Here's how the part is built. I have some questions about the finished solid (model axes, mm). A direction names the side the tool comes from. Round coordinates to 2 decimals unless told otherwise and drop trailing zeros. Loops run counter-clockwise (first coordinate to the right, second up) from the corner with the lowest first, then second, coordinate; pieces in that order, holes last. Notation, with made-up numbers: (36, -32) - (64, -32) arc R9 ccw to (64, -23) - close; hole circle Ø2 at (-1.75, -30). An arc over 180 degrees is marked (long way). Answer as a JSON object with one key per item and string values. Group by question number.
1) I want a section at C-C, the plane x = -12.5. Give the number of separate pieces and of enclosed holes in the cut face, then the cut area to 3 significant figures.
2) Which directions (+Z, -Z, +X, -X, +Y, -Y) give clear straight access to the entire face, cutting with the end or side of a thin tool? Please do faces 1 (the face through (-0.1, 19.4, 0)), 2 (the face through (0, 19, 123)).
3) I want a section at B-B, the plane z = 70. Please give me the cut outline in (x, y), then the cut area to 3 significant figures.
4) If we mould it in two halves opening along X, with no side actions, what happens to faces 3 (the face through (20, 0, 123)), 4 (the face through (0, 20, 123)), 5 (the face through (19, 0, 123))? For each: pulls with the +X half, pulls with the -X half, needs draft (parallel to the pull), parting line crosses it, or undercut.
5) Will this pin go through, and if not, where does the flat tip stop? P1, Ø0.8, axis at x = -7, y = -19.5, coming from the +Z side.
6) If I drill on line 1 along Y through (x, z) = (-16.5, 107); line 2 along Y through (x, z) = (-8.5, 90), over which ranges is the centre line in solid material (lowest first)? Write a range as [from, to].
7) I want a section at A-A, the plane y = -13.5. Please give me the cut outline in (x, z).
from build123d import *

# Parameters (mm, degrees)
F0_W     = 40
F0_H     = 40
F0_W_2   = 38
F0_H_2   = 38
F1_DEPTH = 250
F2_W     = 30
F2_H     = 5
F3_DEPTH = 25


with BuildPart() as f1:
    # F0 (on Top) → F1 (new body)
    with BuildSketch(Plane.XY):
        Rectangle(F0_W, F0_H)
        Rectangle(F0_W_2, F0_H_2, mode=Mode.SUBTRACT)
    extrude(amount=F1_DEPTH)

    # F2 (on face) → F3 (cut)
    with BuildSketch(Plane.XZ.offset(20)):
        Rectangle(F2_W, F2_H)
        with Locations((0, 10)):
            Rectangle(F2_W, F2_H)
        with Locations((0, 20)):
            Rectangle(F2_W, F2_H)
        with Locations((0, 30)):
            Rectangle(F2_W, F2_H)
        with Locations((0, 40)):
            Rectangle(F2_W, F2_H)
        with Locations((0, 50)):
            Rectangle(F2_W, F2_H)
        with Locations((0, 60)):
            Rectangle(F2_W, F2_H)
        with Locations((0, 70)):
            Rectangle(F2_W, F2_H)
        with Locations((0, 80)):
            Rectangle(F2_W, F2_H)
        with Locations((0, 90)):
            Rectangle(F2_W, F2_H)
        with Locations((0, 100)):
            Rectangle(F2_W, F2_H)
        with Locations((0, 110)):
            Rectangle(F2_W, F2_H)
        with Locations((0, 120)):
            Rectangle(F2_W, F2_H)
        with Locations((0, 130)):
            Rectangle(F2_W, F2_H)
        with Locations((0, 140)):
            Rectangle(F2_W, F2_H)
        with Locations((0, 150)):
            Rectangle(F2_W, F2_H)
        with Locations((0, 160)):
            Rectangle(F2_W, F2_H)
        with Locations((0, 170)):
            Rectangle(F2_W, F2_H)
        with Locations((0, 180)):
            Rectangle(F2_W, F2_H)
        with Locations((0, 190)):
            Rectangle(F2_W, F2_H)
        with Locations((0, 200)):
            Rectangle(F2_W, F2_H)
        with Locations((0, 210)):
            Rectangle(F2_W, F2_H)
        with Locations((0, 220)):
            Rectangle(F2_W, F2_H)
        with Locations((0, 230)):
            Rectangle(F2_W, F2_H)
        with Locations((0, 240)):
            Rectangle(F2_W, F2_H)
        with Locations((0, 250)):
            Rectangle(F2_W, F2_H)
        with Locations((0, 260)):
            Rectangle(F2_W, F2_H)
        with Locations((0, 270)):
            Rectangle(F2_W, F2_H)
        with Locations((0, 280)):
            Rectangle(F2_W, F2_H)
        with Locations((0, 290)):
            Rectangle(F2_W, F2_H)
    extrude(amount=-F3_DEPTH, mode=Mode.SUBTRACT)


solid = f1.part
Outcome:
{
 "1": {"separate pieces": "26", "enclosed holes": "0", "area": "375 mm^2"},
 "2": {"face 1": "-Z, +X, -X, +Y, -Y", "face 2": "+Z, -Z"},
 "3": {"outline": "(-20, -20) - (-15, -20) - (-15, -19) - (-19, -19) - (-19, 19) - (19, 19) - (19, -19) - (15, -19) - (15, -20) - (20, -20) - (20, 20) - (-20, 20) - close", "area": "126 mm^2"},
 "4": {"face 3": "pulls with the +X half", "face 4": "needs draft", "face 5": "undercut"},
 "5": {"P1": "z = 247.5"},
 "6": {"line 1": "[-20, -19], [19, 20]", "line 2": "[19, 20]"},
 "7": {"outline": "(-20, 0) - (-19, 0) - (-19, 250) - (-20, 250) - close; (19, 0) - (20, 0) - (20, 250) - (19, 250) - close"}
}
